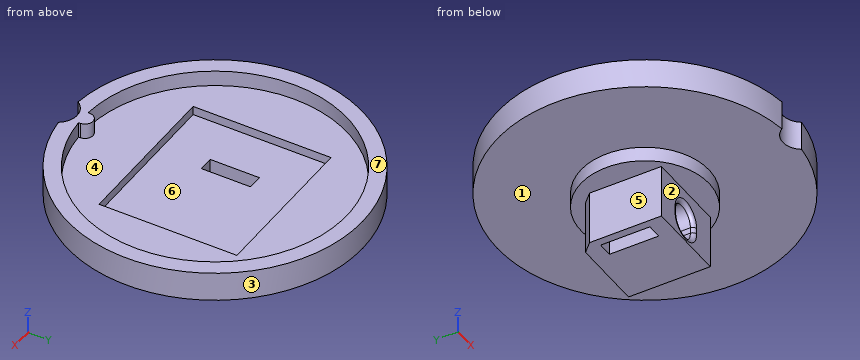
from build123d import *

# Parameters (mm, degrees)
SKETCH012_R     = 15
PAD002_DEPTH    = 3
POCKET004_DEPTH = 1.6
SKETCH013_W     = 16
SKETCH013_H     = 14
POCKET005_DEPTH = 2.5
PAD003_DEPTH    = 7
SKETCH015_R     = 6.5
PAD004_DEPTH    = 1.5
SKETCH016_W     = 1.5
SKETCH016_H     = 5
POCKET006_DEPTH = 10.001
POCKET013_DEPTH = 10.001
POCKET015_DEPTH = 34.90725
FILLET_R        = 0.4
FILLET002_R     = 0.4


with BuildPart() as part:
    # Sketch012 → Pad002 (new body)
    with BuildSketch(Plane.XY):
        with Locations((-60, -20)):
            Circle(SKETCH012_R)
    extrude(amount=-PAD002_DEPTH)

    # Sketch011 → Pocket004 (cut)
    with BuildSketch(Plane.XY):
        with BuildLine():
            ThreePointArc((-59.190336, -33.176677), (-60, -32.39), (-60.809664, -33.176677))
            Line((-60.809664, -33.176677), (-60.821837, -33.374774))
            ThreePointArc((-59.178163, -33.374774), (-60, -6.6), (-60.821837, -33.374774))
            Line((-59.178163, -33.374774), (-59.190336, -33.176677))
        make_face()
    extrude(amount=-POCKET004_DEPTH, mode=Mode.SUBTRACT)

    # Sketch013 → Pocket005 (cut)
    with BuildSketch(Plane.XY):
        with Locations((-60, -20)):
            Rectangle(SKETCH013_W, SKETCH013_H)
    extrude(amount=-POCKET005_DEPTH, mode=Mode.SUBTRACT)

    # Sketch014 → Pad003 (join)
    with BuildSketch(Plane.XY.offset(-3)):
        Polygon((-64.15, -24.15), (-55.85, -24.15), (-55.85, -15.85), (-63.150934, -15.85), (-64.15, -16.849066), align=None)
    extrude(amount=-PAD003_DEPTH)

    # Sketch015 → Pad004 (join)
    with BuildSketch(Plane.XY.offset(-3)):
        with Locations((-60, -20)):
            Circle(SKETCH015_R)
    extrude(amount=-PAD004_DEPTH)

    # Sketch016 → Pocket006 (cut, through all)
    with BuildSketch(Plane.XY):
        with Locations((-62.6, -20)):
            Rectangle(SKETCH016_W, SKETCH016_H)
    extrude(amount=-POCKET006_DEPTH, mode=Mode.SUBTRACT)

    # Sketch025 → Pocket013 (cut, through all)
    with BuildSketch(Plane.XY):
        with BuildLine():
            ThreePointArc((-58.325571, -34.90625), (-60, -34), (-61.674429, -34.90625))
            ThreePointArc((-61.674429, -34.90625), (-60, -35), (-58.325571, -34.90625))
        make_face()
    extrude(amount=-POCKET013_DEPTH, mode=Mode.SUBTRACT)

    # Sketch028 → Pocket015 (cut, through all)
    with BuildSketch(Plane.XZ):
        with BuildLine():
            Line((-58.56, -7.35), (-58.56, -7.95))
            ThreePointArc((-61.44, -7.95), (-60, -9.39), (-58.56, -7.95))
            Line((-61.44, -7.35), (-61.44, -7.95))
            ThreePointArc((-58.56, -7.35), (-60, -5.91), (-61.44, -7.35))
        make_face()
    extrude(amount=POCKET015_DEPTH, mode=Mode.SUBTRACT)

    # Fillet
    fillet_edges = [part.edges().sort_by_distance(p)[0] for p in [
        (-58.56, -24.15, -7.65),
    ]]
    fillet(fillet_edges, radius=FILLET_R)

    # Fillet002
    fillet002_edges = [part.edges().sort_by_distance(p)[0] for p in [
        (-58.56, -15.85, -7.65),
    ]]
    fillet(fillet002_edges, radius=FILLET002_R)


with BuildPart() as part_1:
    # Body001 placement: moved
    add(part.part.moved(Location((60, 20, 1.6))))


solid = part_1.part
Check sheet for the modelled part. Datum: model origin and axes. Units: mm. Face numbers are marked on the shaded views. A direction names the side the tool comes from. Give positions to 0.01 mm unless a question says otherwise; leave off trailing zeros. Loops run counter-clockwise (first coordinate to the right, second up) from the corner with the lowest first, then second, coordinate; pieces in that order, holes last. Notation, with made-up numbers: M 19,2.25 L 25,2.25 A20 ccw 25,20.25 Z; hole C 55,-16.5 d9. An arc over 180 degrees is marked long. Return JSON: item names as keys, results as strings. Group by question number.
1. Cross-section at C-C on x = -13. Record the boundary of the cut face in (y, z).
2. Mould release check, pull along X, two halves, no side actions. Record for the marked faces 4, 5, 6 and 7: released by +X, released by -X, zero draft, split by the parting line, or undercut.
3. Cross-section at A-A on y = 0. Record the boundary of the cut face in (x, z), plus the area to 3 significant figures.
4. Cross-section at B-B on x = 0. Record the boundary of the cut face in (y, z).
5. Tool access check on the marked faces 1, 2 and 3. Record the directions out of +Z, -Z, +X, -X, +Y, -Y that give a thin tool (end or side, any length) a straight path to the whole face; none if there is none.
6. Thickness scan on L1, parallel to X at y = 0, z = 1.2; L2, parallel to Z at x = 7, y = 9; L3, parallel to X at y = -4, z = -3.25. Record the ranges inside material, lowest first.
7. Go/stop test with flat-tipped pins: pin 1 (1.5 mm diameter, centred on y = -1, z = -3.5, fed in from -X); pin 2 (1.2 mm diameter, centred on x = -2.5, z = -6, fed in from +Y); pin 3 (6 mm diameter, centred on x = 1.5, z = -4.5, fed in from -Y). Record where each tip stops, or that it passes through.
Return value:
{
 "1": {"outline": "M -7.48,-1.4 L 7.48,-1.4 L 7.48,1.6 L 3.25,1.6 L 3.25,0 L -3.25,0 L -3.25,1.6 L -7.48,1.6 Z"},
 "2": {"face 4": "undercut", "face 5": "released by -X", "face 6": "undercut", "face 7": "zero draft"},
 "3": {"outline": "M -15,-1.4 L -6.5,-1.4 L -6.5,-2.9 L -4.15,-2.9 L -4.15,-8.4 L -3.35,-8.4 L -3.35,-0.9 L -8,-0.9 L -8,0 L -13.4,0 L -13.4,1.6 L -15,1.6 Z; M -1.85,-8.4 L 4.15,-8.4 L 4.15,-2.9 L 6.5,-2.9 L 6.5,-1.4 L 15,-1.4 L 15,1.6 L 13.4,1.6 L 13.4,0 L 8,0 L 8,-0.9 L -1.85,-0.9 Z; hole M -1.44,-6.35 A1.44 ccw 1.44,-6.35 L 1.44,-5.75 A1.44 ccw -1.44,-5.75 Z", "area": "78.4 mm^2"},
 "4": {"outline": "M -14,-1.4 L -6.5,-1.4 L -6.5,-2.9 L -4.15,-2.9 L -4.15,-3.91 A0.4 ccw -3.75,-4.31 L 3.75,-4.31 A0.4 ccw 4.15,-3.91 L 4.15,-2.9 L 6.5,-2.9 L 6.5,-1.4 L 15,-1.4 L 15,1.6 L 13.4,1.6 L 13.4,0 L 7,0 L 7,-0.9 L -7,-0.9 L -7,0 L -12.39,0 L -12.39,1.6 L -14,1.6 Z; M -4.15,-8.4 L 4.15,-8.4 L 4.15,-8.19 A0.4 ccw 3.75,-7.79 L -3.75,-7.79 A0.4 ccw -4.15,-8.19 Z"},
 "5": {"face 1": "-Z", "face 2": "-Z, +X, -X, -Y", "face 3": "+Z, -Z"},
 "6": {"L1": "-15 to -13.4, 13.4 to 15", "L2": "-1.4 to 0", "L3": "-4.15 to 4.15"},
 "7": {"pin 1": "x = -6.48", "pin 2": "y = 4.15", "pin 3": "y = -6.5"}
}
